```python
from build123d import *

# Parameters (mm, degrees)
F0_W     = 127
F0_H     = 273.558
F0_H_2   = 431.8
F0_R     = 101.6
F0_H_3   = 152.4
F0_W_2   = 1397
F1_DEPTH = 203.2
F2_DEPTH = 838.2
F4_R     = 127


with BuildPart() as f1:
    # F0 (on Front) → F1 (new body)
    with BuildSketch(Plane.XZ):
        with Locations((216.0754676017, 341.5033780212)):
            Rectangle(F0_W, F0_H)
        with Locations((216.0754676017, -11.1756219788)):
            Rectangle(F0_W, F0_H_2)
        with BuildLine():
            Line((1422.5754676017, 204.7243780212), (279.5754676017, 204.7243780212))
            Line((279.5754676017, 204.7243780212), (279.5754676017, -227.0756219788))
            Line((279.5754676017, -227.0756219788), (1676.5754676017, -227.0756219788))
            Line((1676.5754676017, -227.0756219788), (1676.5754676017, -49.2756219788))
            ThreePointArc((1676.5754676017, -49.2756219788), (1602.1805900231, 130.3295004426), (1422.5754676017, 204.7243780212))
        make_face()
        with Locations((1422.5754676017, -49.2756219788)):
            Circle(F0_R, mode=Mode.SUBTRACT)
        with Locations((216.0754676017, -303.2756219788)):
            Rectangle(F0_W, F0_H_3)
        with Locations((978.0754676017, -303.2756219788)):
            Rectangle(F0_W_2, F0_H_3)
        with Locations((216.0754676017, -595.3756219788)):
            Rectangle(F0_W, F0_H_2)
        with BuildLine():
            Line((1676.5754676017, -379.4756219788), (279.5754676017, -379.4756219788))
            Line((279.5754676017, -379.4756219788), (279.5754676017, -811.2756219788))
            Line((279.5754676017, -811.2756219788), (1422.5754676017, -811.2756219788))
            ThreePointArc((1422.5754676017, -811.2756219788), (1602.1805900231, -736.8807444001), (1676.5754676017, -557.2756219788))
            Line((1676.5754676017, -557.2756219788), (1676.5754676017, -379.4756219788))
        make_face()
        with Locations((1422.5754676017, -557.2756219788)):
            Circle(F0_R, mode=Mode.SUBTRACT)
        Polygon((279.5754676017, -811.2756219788), (152.5754676017, -811.2756219788), (152.5754676017, -1084.8336219788), (277.5078122768, -1084.8336219788), align=None)
    extrude(amount=F1_DEPTH)

    # F0 (on Front) → F2 (join)
    with BuildSketch(Plane.XZ):
        Polygon((279.5754676017, -811.2756219788), (152.5754676017, -811.2756219788), (152.5754676017, -1084.8336219788), (277.5078122768, -1084.8336219788), align=None)
        with Locations((216.0754676017, -595.3756219788)):
            Rectangle(F0_W, F0_H_2)
        with Locations((216.0754676017, -303.2756219788)):
            Rectangle(F0_W, F0_H_3)
        with Locations((216.0754676017, -11.1756219788)):
            Rectangle(F0_W, F0_H_2)
        with Locations((216.0754676017, 341.5033780212)):
            Rectangle(F0_W, F0_H)
    extrude(amount=F2_DEPTH)

    # F4
    f4_edges = [f1.edges().sort_by_distance(p)[0] for p in [
        (216.075468, -838.2, 478.282378),
        (215.04164, -838.2, -1084.833622),
    ]]
    fillet(f4_edges, radius=F4_R)


solid = f1.part
```
Part model, mm, in its own coordinate system. A direction names the side the tool comes from. Coordinates: 2 decimals unless noted, no trailing zeros. Order: outer loops, then holes, each group sorted by start corner. A loop starts at its lowest first (then second) coordinate and runs counter-clockwise, first axis right, second up. Notation, with made-up numbers: (70, 59) -> (103, 59) arc R29 cw to (103, 88) -> close; hole circle Ø5 at (43.5, 47.25). An arc over 180 degrees is marked (long way). Put each result on its own line as item: value. Start each with the question number.
(1) Probe line 1 along Y through (x, z) = (295.5, -85.5); line 2 along X through (y, z) = (-288, -523); line 3 along Z through (x, y) = (721, -135). List the from-to ranges inside material, lowest first. Write a range as [from, to].
(2) Mould opens along Z. For faces 6 (the face through (1321.074, -100.178, -552.808)), 7 (the face through (152.575, -413, -292)), 8 (the face through (214, -351, -1084.834)) say: pulls with the +Z half, pulls with the -Z half, needs draft (parallel to the pull), parting line crosses it, or undercut.
(3) Which spindle directions (+Z, -Z, +X, -X, +Y, -Y) get a long thin tool onto all of the face, cutting with end or side? Do faces 1 (the face through (968, -203.2, -296)), 2 (the face through (843, -100, -811.276)), 3 (the face through (859, -100, 204.724)), 4 (the face through (215, -351, 478.282)), 5 (the face through (1676.575, -100, -307)). Say none if no direction does.
(4) Band-saw the part on C-C (x = 1390.5). Give the cut face in (y, z).
(5) Band-saw the part on D-D (y = -625.5). Give the cut face in (x, z), then the cut area to 3 significant figures.
(6) Band-saw the part on B-B (z = -593). Give the cut face in (x, y), then the cut area to 3 significant figures.
(7) Band-saw the part on A-A (y = -167). Give the cut face in (x, z), then the cut area to 3 significant figures.
(8) Pin check, flat tips, straight feed: pin 1 Ø12 at (x, y) = (1252, -180.5) entering from -Z; pin 2 Ø2 at (y, z) = (-432.5, -752) entering from +X. Stop position of each tip, or through.
Determined:
1. line 1: y = [-203.2, 0]
1. line 2: x = [152.58, 279.58]
1. line 3: z = [-811.28, 204.72]
2. face 6: undercut
2. face 7: needs draft
2. face 8: pulls with the -Z half
3. face 1: +Z, -Z, +X, -Y
3. face 2: -Z, +X, +Y, -Y
3. face 3: +Z, +X, +Y, -Y
3. face 4: +Z, +X, -X, +Y, -Y
3. face 5: +Z, -Z, +X, +Y, -Y
4. outline: (-203.2, -811.28) -> (0, -811.28) -> (0, -653.68) -> (-203.2, -653.68) -> close; (-203.2, -460.87) -> (0, -460.87) -> (0, -145.68) -> (-203.2, -145.68) -> close; (-203.2, 47.13) -> (0, 47.13) -> (0, 204.72) -> (-203.2, 204.72) -> close
5. outline: (152.58, -1084.83) -> (277.51, -1084.83) -> (279.58, -811.28) -> (279.58, 478.28) -> (152.58, 478.28) -> close
5. area: 198,000 mm²
6. outline: (152.58, -838.2) -> (279.58, -838.2) -> (279.58, -203.2) -> (1327.46, -203.2) -> (1327.46, 0) -> (152.58, 0) -> close; (1517.69, -203.2) -> (1674.05, -203.2) -> (1674.05, 0) -> (1517.69, 0) -> close
6. area: 351,000 mm²
7. outline: (152.58, -1084.83) -> (277.51, -1084.83) -> (279.58, -811.28) -> (1422.58, -811.28) arc R254 ccw to (1676.58, -557.28) -> (1676.58, -49.28) arc R254 ccw to (1422.58, 204.72) -> (279.58, 204.72) -> (279.58, 478.28) -> (152.58, 478.28) -> close; hole circle Ø203.2 at (1422.58, -557.28); hole circle Ø203.2 at (1422.58, -49.28)
7. area: 1,530,000 mm²
8. pin 1: stops at z = -811.28
8. pin 2: stops at x = 279.58
